Geometry: final body of the model. Coordinates: model frame, mm. Face numbers are marked on the shaded views. A direction names the side the tool comes from. Round coordinates to 2 decimals unless told otherwise and drop trailing zeros. Order: outer loops, then holes, each group sorted by start corner. A loop starts at its lowest first (then second) coordinate and runs counter-clockwise, first axis right, second up. Notation, with made-up numbers: M 32,-29.5 L 53,-29.5 A7 ccw 53,-16.5 Z; hole C -34,-16 d1. An arc over 180 degrees is marked long. Put each result on its own line as item: value. Start each with the question number.
1) Material intervals for probe 1 along Y at (x, z) = (-42, 0.75); probe 2 along Z at (x, y) = (29.5, 190); probe 3 along X at (y, z) = (198.5, 9), sorted ascending. Write a range as [from, to].
2) Access query for the marked faces 1 and 2. Directions: +Z, -Z, +X, -X, +Y, -Y. A direction counts if a zero-diameter tool reaches every point of the face in a straight line with its end or side. Return the directions, or none.
3) Section B-B, the plane y = 214. Return loops of the section in (x, z), then the cut area to 3 significant figures.
4) First-contact query: P1, Ø4, axis at x = -104.94, y = 231.51, coming from the +Z side; P2, Ø4, axis at y = 193, z = 4.5, coming from the +X side; P3, Ø5, axis at x = -95.5, y = 222.5, coming from the +Z side; P4, Ø2, axis at x = -89.5, z = 8.5, coming from the +Y side. Flat tips, straight axial feed; report the tip coordinate or a pass-through.
5) Section C-C, the plane z = 2.5. Return loops of the section in (x, y), then the cut area to 3 significant figures.
6) Section A-A, the plane x = -12. Return loops of the section in (y, z).
7) Section D-D, the plane x = -36.5. Return loops of the section in (y, z).
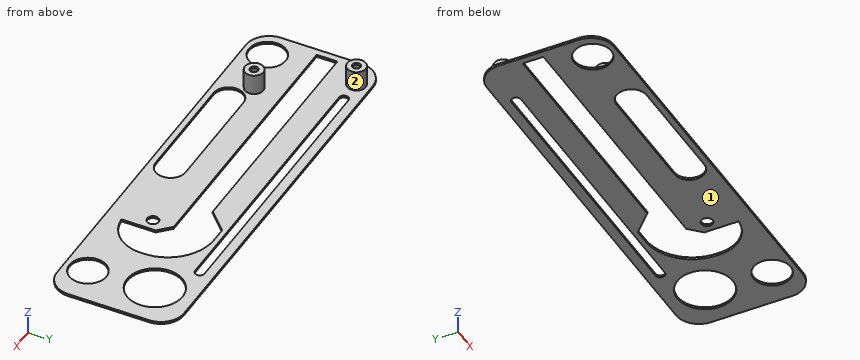
from build123d import *

# Parameters (mm, degrees)
SKETCH001_W   = 178
SKETCH001_H   = 55
SKETCH001_R   = 2.5
SKETCH001_R_2 = 8
SKETCH001_R_3 = 12.004096
PAD_DEPTH     = 1
SKETCH003_R   = 4
PAD001_DEPTH  = 9
SKETCH004_R   = 1.3
POCKET_DEPTH  = 9
FILLET_R      = 10
FILLET001_R   = 10
CHAMFER_SIZE  = 0.5


with BuildPart() as part:
    # Sketch001 → Pad (new body)
    with BuildSketch(Plane.XY):
        with Locations((-27.95005, 210.084131)):
            Rectangle(SKETCH001_W, SKETCH001_H)
        with Locations((5.54995, 200.560838)):
            Circle(SKETCH001_R, mode=Mode.SUBTRACT)
        with Locations((-105.249172, 192.692063)):
            Circle(SKETCH001_R_2, mode=Mode.SUBTRACT)
        with Locations((44.750828, 192.692063)):
            Circle(SKETCH001_R_2, mode=Mode.SUBTRACT)
        with Locations((42.270485, 220.407623)):
            Circle(SKETCH001_R_3, mode=Mode.SUBTRACT)
        with BuildLine():
            ThreePointArc((25.54995, 206.028969), (20.061493, 220.835101), (5.54995, 227.060838))
            Line((-1.19441, 227.060838), (5.54995, 227.060838))
            Line((-9.694456, 218.560838), (-1.19441, 227.060838))
            Line((-113.95005, 218.561117), (-9.694456, 218.560838))
            Line((-113.95005, 218.561117), (-113.95005, 209.560838))
            Line((-113.95005, 209.560838), (-9.618024, 209.560838))
            Line((-9.618024, 209.560838), (5.54995, 209.560838))
            Line((5.54995, 209.560838), (10.697892, 204.412896))
            Line((10.697892, 189.560838), (10.697892, 204.412896))
            ThreePointArc((10.697892, 189.560838), (21.441031, 194.803313), (25.54995, 206.028969))
        make_face(mode=Mode.SUBTRACT)
        with BuildLine():
            ThreePointArc((-74.793427, 198.14003), (-81.282837, 191.65062), (-74.793427, 185.16121))
            Line((-74.793427, 185.16121), (-26.440948, 185.16121))
            ThreePointArc((-26.440948, 185.16121), (-19.951538, 191.65062), (-26.440948, 198.14003))
            Line((-74.793427, 198.14003), (-26.440948, 198.14003))
        make_face(mode=Mode.SUBTRACT)
        with BuildLine():
            ThreePointArc((-94.612823, 233.364261), (-96.6561, 231.320984), (-94.612823, 229.277707))
            Line((-94.612823, 229.277707), (25.728859, 229.277707))
            ThreePointArc((25.728859, 229.277707), (27.772136, 231.320984), (25.728859, 233.364261))
            Line((-94.612823, 233.364261), (25.728859, 233.364261))
        make_face(mode=Mode.SUBTRACT)
    extrude(amount=PAD_DEPTH)

    # Sketch003 (on Face28 of Pad) → Pad001 (join)
    with BuildSketch(Plane.XY.offset(1)):
        with Locations((-84.923561, 197.527756)):
            Circle(SKETCH003_R)
        with Locations((-104.933395, 231.507965)):
            Circle(SKETCH003_R)
    extrude(amount=PAD001_DEPTH)

    # Sketch004 (on Face31 of Pad001) → Pocket (cut)
    with BuildSketch(Plane.XY.offset(10)):
        with Locations((-84.917816, 197.526398)):
            Circle(SKETCH004_R)
        with Locations((-104.937256, 231.505722)):
            Circle(SKETCH004_R)
    extrude(amount=-POCKET_DEPTH, mode=Mode.SUBTRACT)

    # Fillet
    fillet_edges = [part.edges().sort_by_distance(p)[0] for p in [
        (-116.95005, 182.584131, 0.5),
        (61.04995, 182.584131, 0.5),
    ]]
    fillet(fillet_edges, radius=FILLET_R)

    # Fillet001
    fillet001_edges = [part.edges().sort_by_distance(p)[0] for p in [
        (61.04995, 237.584131, 0.5),
        (-116.95005, 237.584131, 0.5),
    ]]
    fillet(fillet001_edges, radius=FILLET001_R)

    # Chamfer
    chamfer_edges = [part.edges().sort_by_distance(p)[0] for p in [
        (-106.237256, 231.505722, 10),
        (-86.217816, 197.526398, 10),
    ]]
    chamfer(chamfer_edges, length=CHAMFER_SIZE)


solid = part.part
Result sheet:
1. probe 1: y = [182.58, 185.16], [198.14, 209.56], [218.56, 229.28], [233.36, 237.58]
1. probe 2: z = [0, 1]
1. probe 3: x = [-88.8, -85.78], [-84.06, -81.04]
2. face 1: -Z, +X, -X, +Y, -Y
2. face 2: +Z
3. outline: M -116.95,0 L -113.95,0 L -113.95,1 L -116.95,1 Z; M 24.33,0 L 32.12,0 L 32.12,1 L 24.33,1 Z; M 52.42,0 L 61.05,0 L 61.05,1 L 52.42,1 Z
3. area: 19.4 mm2
4. P1: stops at z = 10
4. P2: stops at x = -81.82
4. P3: stops at z = 1
4. P4: stops at y = 199.32
5. outline: C -104.93,231.51 d8; C -84.92,197.53 d8; hole C -104.94,231.51 d2.6; hole C -84.92,197.53 d2.6
5. area: 89.9 mm2
6. outline: M 182.58,0 L 209.56,0 L 209.56,1 L 182.58,1 Z; M 218.56,0 L 229.28,0 L 229.28,1 L 218.56,1 Z; M 233.36,0 L 237.58,0 L 237.58,1 L 233.36,1 Z
7. outline: M 182.58,0 L 185.16,0 L 185.16,1 L 182.58,1 Z; M 198.14,0 L 209.56,0 L 209.56,1 L 198.14,1 Z; M 218.56,0 L 229.28,0 L 229.28,1 L 218.56,1 Z; M 233.36,0 L 237.58,0 L 237.58,1 L 233.36,1 Z
